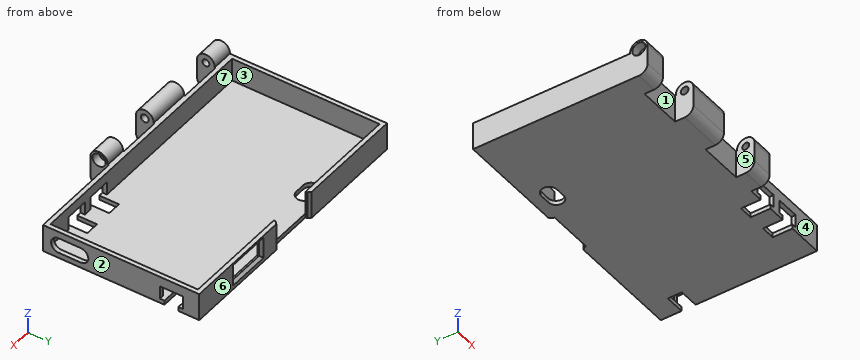
```python
from build123d import *

# Parameters (mm, degrees)
SKETCH035_R     = 1.6
PAD_DEPTH       = 61.5
PAD_DEPTH_BACK  = 61.5
SKETCH037_W     = 8.4
SKETCH037_H     = 43
SKETCH037_H_2   = 20
POCKET007_DEPTH = 17.001
SKETCH038_R     = 3
POCKET008_DEPTH = 4
SKETCH039_R     = 3
POCKET009_DEPTH = 4
SKETCH041_W     = 67.4
SKETCH041_H     = 119
POCKET011_DEPTH = 11
POCKET012_DEPTH = 2
SKETCH043_W     = 7.5
SKETCH043_H     = 17.6
SKETCH043_W_2   = 15
SKETCH043_H_2   = 20.8
POCKET013_DEPTH = 2
POCKET014_DEPTH = 9
POCKET015_DEPTH = 9
CHAMFER_SIZE    = 1.2
SKETCH062_R     = 1.8
POCKET020_DEPTH = 20
SKETCH071_W     = 71.8
SKETCH071_H     = 123
POCKET026_DEPTH = 0.4


with BuildPart() as part:
    # Sketch035 → Pad (new body, two sides)
    with BuildSketch(Plane.YZ) as pad_sk:
        with BuildLine():
            Line((75.8, 0), (75.8, -13))
            Line((75.8, -13), (0, -13))
            ThreePointArc((-4, -9), (-2.828427, -11.828427), (0, -13))
            Line((-4, 0), (-4, -9))
            ThreePointArc((4, 0), (0, 4), (-4, 0))
            Line((4, 0), (4.4, 0))
            Line((4.4, 0), (75.8, 0))
        make_face()
        Circle(SKETCH035_R, mode=Mode.SUBTRACT)
    extrude(amount=PAD_DEPTH)
    extrude(pad_sk.sketch, amount=-PAD_DEPTH_BACK)

    # Sketch037 (on Face4 of Pad) → Pocket007 (cut, through all)
    with BuildSketch(Plane.YX.offset(13)):
        with Locations((0.2, 40)):
            Rectangle(SKETCH037_W, SKETCH037_H)
        with Locations((0.2, -1.5)):
            Rectangle(SKETCH037_W, SKETCH037_H_2)
        with Locations((0.2, -41.5)):
            Rectangle(SKETCH037_W, SKETCH037_H_2)
    extrude(amount=-POCKET007_DEPTH, mode=Mode.SUBTRACT)

    # Sketch038 (on Face22 of Pocket007) → Pocket008 (cut)
    with BuildSketch(Plane.YZ.offset(18.5)):
        Circle(SKETCH038_R)
    extrude(amount=-POCKET008_DEPTH, mode=Mode.SUBTRACT)

    # Sketch039 (on Face2 of Pocket008) → Pocket009 (cut)
    with BuildSketch(Plane(origin=(-61.5, 0, 0), x_dir=(0, 1, 0), z_dir=(-1, 0, 0))):
        Circle(SKETCH039_R)
    extrude(amount=-POCKET009_DEPTH, mode=Mode.SUBTRACT)

    # Sketch041 (on Face3 of Pocket009) → Pocket011 (cut)
    with BuildSketch(Plane(origin=(0, 0, 0), x_dir=(0, -1, 0), z_dir=(0, 0, 1))):
        with Locations((-40.1, 0)):
            Rectangle(SKETCH041_W, SKETCH041_H)
    extrude(amount=-POCKET011_DEPTH, mode=Mode.SUBTRACT)

    # Sketch042 (on Face31 of Pocket011) → Pocket012 (cut)
    with BuildSketch(Plane(origin=(0, 0, -11), x_dir=(0, -1, 0), z_dir=(0, 0, 1))):
        with BuildLine():
            ThreePointArc((-63.6, -19.6), (-67.1, -16.1), (-70.6, -19.6))
            Line((-70.6, -19.6), (-70.6, -24.1))
            ThreePointArc((-70.6, -24.1), (-67.1, -27.6), (-63.6, -24.1))
            Line((-63.6, -19.6), (-63.6, -24.1))
        make_face()
    extrude(amount=-POCKET012_DEPTH, mode=Mode.SUBTRACT)

    # Sketch043 (on Face7 of Pocket012) → Pocket013 (cut)
    with BuildSketch(Plane.ZX.offset(75.8)):
        with Locations((-6.25, 29.3)):
            Rectangle(SKETCH043_W, SKETCH043_H)
        with Locations((-5.5, -0.6)):
            Rectangle(SKETCH043_W_2, SKETCH043_H_2)
    extrude(amount=-POCKET013_DEPTH, mode=Mode.SUBTRACT)

    # Sketch044 (on Face19 of Pocket013) → Pocket014 (cut)
    with BuildSketch(Plane.YZ.offset(61.5)):
        with BuildLine():
            ThreePointArc((11.6, -3.5), (8.1, -7), (11.6, -10.5))
            Line((11.6, -10.5), (21.6, -10.5))
            ThreePointArc((21.6, -10.5), (25.1, -7), (21.6, -3.5))
            Line((11.6, -3.5), (21.6, -3.5))
        make_face()
        Polygon((57.8, -5), (68.4, -5), (68.4, -11), (66.3, -11), (66.3, -13), (59.9, -13), (59.9, -11), (57.8, -11), align=None)
    extrude(amount=-POCKET014_DEPTH, mode=Mode.SUBTRACT)

    # Sketch045 (on Face20 of Pocket014) → Pocket015 (cut)
    with BuildSketch(Plane(origin=(0, 4.4, 0), x_dir=(0, 0, -1), z_dir=(0, -1, 0))):
        Polygon((5, 33.1), (5, 22.5), (11, 22.5), (11, 24.6), (13, 24.6), (13, 31), (11, 31), (11, 33.1), align=None)
        Polygon((5, 36.9), (11, 36.9), (11, 39), (13, 39), (13, 45.4), (11, 45.4), (11, 47.5), (5, 47.5), align=None)
    extrude(amount=-POCKET015_DEPTH, mode=Mode.SUBTRACT)

    # Chamfer
    chamfer_edges = [part.edges().sort_by_distance(p)[0] for p in [
        (9.8, 75.8, -6.5),
        (-11, 75.8, -6.5),
        (38.1, 75.8, -6.25),
        (29.3, 75.8, -2.5),
        (20.5, 75.8, -6.25),
        (29.3, 75.8, -10),
    ]]
    chamfer(chamfer_edges, length=CHAMFER_SIZE)

    # Sketch062 (on Face29 of Chamfer) → Pocket020 (cut)
    with BuildSketch(Plane(origin=(-31.5, 0, 0), x_dir=(0, 1, 0), z_dir=(-1, 0, 0))):
        Circle(SKETCH062_R)
    extrude(amount=-POCKET020_DEPTH, mode=Mode.SUBTRACT)

    # Sketch071 (on Face1 of Pocket020) → Pocket026 (cut)
    with BuildSketch(Plane(origin=(0, 0, 0), x_dir=(0, -1, 0), z_dir=(0, 0, 1))):
        with Locations((-39.9, 0)):
            Rectangle(SKETCH071_W, SKETCH071_H)
    extrude(amount=-POCKET026_DEPTH, mode=Mode.SUBTRACT)


solid = part.part
```
The model under review builds one solid part; all positions refer to its coordinate system, in mm. Face numbers are marked on the shaded views. A direction names the side the tool comes from. Round coordinates to 2 decimals unless told otherwise and drop trailing zeros. Loops run counter-clockwise (first coordinate to the right, second up) from the corner with the lowest first, then second, coordinate; pieces in that order, holes last.
1) Consider section C-C on y = 33.5. State the section outline as (x, z) points.
Values follow:
outline: (-61.5, -13) - (61.5, -13) - (61.5, -0.4) - (59.5, -0.4) - (59.5, -11) - (-59.5, -11) - (-59.5, -0.4) - (-61.5, -0.4) - close
2) Consider section A-A on x = -21.5. State the section outline as (y, z) points, then the cut area to 3 significant figures.
Values follow:
outline: (-4, -9) arc R4 ccw to (0, -13) - (63.6, -13) - (63.6, -11) - (6.4, -11) - (6.4, -0.4) - (4, -0.4) - (4, 0) arc R4 ccw to (-4, 0) - close; (70.6, -13) - (75.8, -13) - (75.8, -0.4) - (73.8, -0.4) - (73.8, -11) - (70.6, -11) - close; hole circle Ø3.6 at (0, 0)
area: 292 mm2
3) Tool access review of the marked faces 5, 6 and 7: name each direction out of +Z, -Z, +X, -X, +Y, -Y from which nothing blocks a thin tool from reaching the whole face with its end or side.
Values follow:
face 5: +Z, -Z, -Y
face 6: +Z, -Z, +X, -X, +Y
face 7: +Z
4) Consider section B-B on y = 17. State the section outline as (x, z) points.
Values follow:
outline: (-61.5, -13) - (61.5, -13) - (61.5, -10.5) - (59.5, -10.5) - (59.5, -11) - (-59.5, -11) - (-59.5, -0.4) - (-61.5, -0.4) - close; (59.5, -3.5) - (61.5, -3.5) - (61.5, -0.4) - (59.5, -0.4) - close
5) The part is to be moulded in two halves that separate along X. For the marked faces 1, 2, 3 and 4, say which applies: pulls with the +X half, pulls with the -X half, needs draft (parallel to the pull), parting line crosses it, or undercut.
Values follow:
face 1: undercut
face 2: pulls with the +X half
face 3: undercut
face 4: needs draft
6) Wall thickness on line 1 along Y through (x, z) = (-13, -7.25); line 2 along X through (y, z) = (54.5, -8.5); line 3 along Y through (x, z) = (-40.5, -8.5): over which ranges is each line inside the solid? List them lowest first.
Values follow:
line 1: y = -4 to 6.4, 73.8 to 75.8
line 2: x = -61.5 to -59.5, 59.5 to 61.5
line 3: y = 4.4 to 6.4, 73.8 to 75.8
7) Clearance check with flat-ended pins moving along their axes: P1, Ø1, axis at x = -2, z = -3.5, coming from the +Y side; P2, Ø1.6, axis at x = 60, y = 61, coming from the -Z side; P3, Ø3, axis at y = 0, z = 0, coming from the +X side; P4, Ø1, axis at x = 59, z = -12, coming from the -Y side. State where each tip first meets the part, or that it passes through.
Values follow:
P1: stops at y = 6.4
P2: stops at z = -5
P3: passes through
P4: stops at y = 4.4
